```python
from build123d import *

# Parameters (mm, degrees)
F0_R      = 35.353158
F1_DEPTH  = 25
F2_R      = 24.193713
F3_DEPTH  = 15
F3_FACE_R = 24.193713
F4_DEPTH  = 25


with BuildPart() as f1:
    # F0 (on Top) → F1 (new body)
    with BuildSketch(Plane.XY):
        with Locations((0, 3.22861)):
            Circle(F0_R)
    extrude(amount=F1_DEPTH)

    # F2 (on face) → F3 (join)
    with BuildSketch(Plane.XY.offset(25)):
        Circle(F2_R)
    extrude(amount=F3_DEPTH)

    # F3_face (on face) → F4 (cut)
    with BuildSketch(Plane.XY.offset(40)):
        Circle(F3_FACE_R)
    extrude(amount=-F4_DEPTH, mode=Mode.SUBTRACT)


solid = f1.part
```
Read the model definition and answer for the solid it produces. Units are mm, in the model's axes. A direction names the side the tool comes from. Coordinates: 2 decimals unless noted, no trailing zeros. Write each loop counter-clockwise with the first axis right and the second up, starting at its lowest first coordinate (ties: lowest second). Pieces come first, ordered by that corner, then holes. Notation, with made-up numbers: (-16, 56.5) -> (41, 56.5) arc R25 ccw to (41, 91.5) -> close; hole circle Ø1 at (-13.5, 28). An arc over 180 degrees is marked (long way). Write item = value, one per line.
(1) Section A-A on x = 0 is taken. Write down the section's boundary in (y, z).
From the geometry:
outline = (-32.12, 0) -> (38.58, 0) -> (38.58, 25) -> (24.19, 25) -> (24.19, 15) -> (-24.19, 15) -> (-24.19, 25) -> (-32.12, 25) -> close
(2) Section B-B on y = 0 is taken. Write down the section's boundary in (x, z), plus the area to 3 significant figures.
From the geometry:
outline = (-35.21, 0) -> (35.21, 0) -> (35.21, 25) -> (24.19, 25) -> (24.19, 15) -> (-24.19, 15) -> (-24.19, 25) -> (-35.21, 25) -> close
area = 1,280 mm2
(3) Section D-D on z = 5 is taken. Write down the section's boundary in (x, y), plus the area to 3 significant figures.
From the geometry:
outline = circle Ø70.71 at (0, 3.23)
area = 3,930 mm2
(4) Section C-C on z = 20.25 is taken. Write down the section's boundary in (x, y), plus the area to 3 significant figures.
From the geometry:
outline = circle Ø70.71 at (0, 3.23); hole circle Ø48.39 at (0, 0)
area = 2,090 mm2
(5) Straight lines are drawn through the part: L1, parallel to Y at x = 0, z = 20.25; L2, parallel to X at y = 29, z = 2; L3, parallel to Z at x = -12, y = 9. For each, find the intervals that lie inside material, in ascending order. Write a range as from..to.
From the geometry:
L1 = -32.12..-24.19, 24.19..38.58
L2 = -24.2..24.2
L3 = 0..15
(6) Which of the six approach directions +Z, -Z, +X, -X, +Y, -Y give full straight-line access (tool end or side, diameter ignored) to faces 4 (the face through (15.2, 19.4, 25)), 5 (the face through (0, 0, 15))?
From the geometry:
face_4 = +Z, +X, -X, +Y, -Y
face_5 = +Z
(7) For a pull along X with two mould halves and no side action, classify faces 1 (the face through (0, 4, 0)), 2 (the face through (-19.2, -14.72, 20.07)), 3 (the face through (-26.06, 27.12, 12.32)) as +X half, -X half, draft (parallel to the pull), parting line (faces both ways), or undercut.
From the geometry:
face_1 = draft
face_2 = undercut
face_3 = parting line
(8) Given pin 1 Ø10 at (y, z) = (-5.5, 15.5) entering from +X; pin 2 Ø6 at (y, z) = (0, 3.5) entering from +X; pin 3 Ø4 at (x, z) = (-9.5, 10) entering from -Y, each flat-ended and moving along its own axis, determine where each tip first touches the part or whether it passes through.
From the geometry:
pin_1 = 35.16
pin_2 = 35.35
pin_3 = -31.32
